Check sheet for the modelled part. Datum: model origin and axes. Units: mm. A direction names the side the tool comes from. Give positions to 0.01 mm unless a question says otherwise; leave off trailing zeros. Order: outer loops, then holes, each group sorted by start corner. A loop starts at its lowest first (then second) coordinate and runs counter-clockwise, first axis right, second up. Notation, with made-up numbers: (-21.5, 15) -> (21.5, 15) arc R20 ccw to (21.5, 54) -> close; hole circle Ø8 at (10.25, 27). An arc over 180 degrees is marked (long way). One line per question, with ' | ' between items.
```python
from build123d import *

# Parameters (mm, degrees)
F1_DEPTH = 50
F3_R     = 3.2
F4_DEPTH = 16.001
F2_W     = 30
F2_H     = 12
F5_DEPTH = 24.001
F6_R     = 5


with BuildPart() as f1:
    # F0 (on Right) → F1 (new body)
    with BuildSketch(Plane.YZ):
        Polygon((0, -8), (0, 0), (-33, 0), (-33, 9.8), (-49, 9.8), (-49, 3.8), (-43, 3.8), (-43, -24), (-33, -24), (-33, -8), align=None)
    extrude(amount=F1_DEPTH)

    # F3 (on face) → F4 (cut, through all)
    with BuildSketch(Plane(origin=(0, -33, 0), x_dir=(-1, 0, 0), z_dir=(0, 1, 0))):
        with Locations((-25, -14)):
            Circle(F3_R)
    extrude(amount=-F4_DEPTH, mode=Mode.SUBTRACT)

    # F2 (on face) → F5 (cut, through all)
    with BuildSketch(Plane.XY):
        with Locations((25, -26)):
            Rectangle(F2_W, F2_H)
    extrude(amount=-F5_DEPTH, mode=Mode.SUBTRACT)

    # F6
    f6_edges = [f1.edges().sort_by_distance(p)[0] for p in [
        (50, 0, -4),
        (0, 0, -4),
        (50, -33, 4.9),
        (0, -33, 4.9),
        (50, -49, 6.8),
        (0, -49, 6.8),
        (50, -38, -24),
        (0, -38, -24),
        (10, -32, -4),
        (40, -32, -4),
        (40, -20, -4),
        (10, -20, -4),
    ]]
    fillet(f6_edges, radius=F6_R)


solid = f1.part
```
Q1. Section check C-C (y = -35). Enter the section's corners in (x, z), and give its area (3 significant figures).
Result sheet:
outline: (0, -19) arc R5 ccw to (5, -24) -> (45, -24) arc R5 ccw to (50, -19) -> (50, 0) -> (49, 0) -> (49, 9.8) -> (1, 9.8) -> (1, 0) -> (0, 0) -> close; hole circle Ø6.4 at (25, -14) | area: 1,630 mm2
Q2. Mould release check, pull along Y, two halves, no side actions. Record for faces 4 (the face through (48, -1, -4)), 5 (the face through (12, -31, -4)), 6 (the face through (1, -38, -22)): pulls with the +Y half, pulls with the -Y half, needs draft (parallel to the pull), parting line crosses it, or undercut.
Result sheet:
face 4: pulls with the +Y half | face 5: undercut | face 6: needs draft
Q3. Section check A-A (x = 30). Enter the section's corners in (y, z), and give its area (3 significant figures).
Result sheet:
outline: (-49, 3.8) -> (-43, 3.8) -> (-43, -24) -> (-33, -24) -> (-33, -8) -> (-32, -8) -> (-32, 0) -> (-33, 0) -> (-33, 9.8) -> (-49, 9.8) -> close; (-20, -8) -> (0, -8) -> (0, 0) -> (-20, 0) -> close | area: 542 mm2
Q4. Depth check by flat-ended pin: pin 1 Ø5 at (x, y) = (32.5, -46) entering from -Z; pin 2 Ø4 at (x, z) = (25, -14) entering from +Y; pin 3 Ø5 at (x, z) = (26.5, -1) entering from -Y; pin 4 Ø17.5 at (x, z) = (29.5, -14.5) entering from +Y. Enter the tip coordinate at first touch or a pass-through.
Result sheet:
pin 1: stops at z = 3.8 | pin 2: passes through | pin 3: stops at y = -43 | pin 4: stops at y = 0
Q5. Access from +Z, -Z, +X, -X, +Y, -Y to the whole of each face (thin tool, end or side, straight path). Record for faces 1 (the face through (25, -43, -10)), 2 (the face through (38, -31, -4)), 3 (the face through (1, -35, 5)).
Result sheet:
face 1: -Z, +X, -X, -Y | face 2: +Z, -Z | face 3: +Z, -X, +Y
Q6. Section check B-B (z = -14). Enter the section's corners in (x, y).
Result sheet:
outline: (0, -43) -> (21.8, -43) -> (21.8, -33) -> (0, -33) -> close; (28.2, -43) -> (50, -43) -> (50, -33) -> (28.2, -33) -> close
Q7. Thickness scan on line 1 (Y direction, x = 15.5, z = -1); line 2 (Z direction, x = 25, y = -36); line 3 (Y direction, x = 27, z = -18). Record the ranges inside material, lowest first.
Result sheet:
line 1: y = -43 to -32, -20 to 0 | line 2: z = -24 to -17.2, -10.8 to 9.8 | line 3: y = -43 to -33
Q8. Section check D-D (x = 25). Enter the section's corners in (y, z), and give its area (3 significant figures).
Result sheet:
outline: (-49, 3.8) -> (-43, 3.8) -> (-43, -10.8) -> (-33, -10.8) -> (-33, -8) -> (-32, -8) -> (-32, 0) -> (-33, 0) -> (-33, 9.8) -> (-49, 9.8) -> close; (-43, -24) -> (-33, -24) -> (-33, -17.2) -> (-43, -17.2) -> close; (-20, -8) -> (0, -8) -> (0, 0) -> (-20, 0) -> close | area: 478 mm2
